Geometry check sheet. Reference: the model listing, model coordinates, mm. A direction names the side the tool comes from. Round coordinates to 2 decimals unless told otherwise and drop trailing zeros. Order: outer loops, then holes, each group sorted by start corner. A loop starts at its lowest first (then second) coordinate and runs counter-clockwise, first axis right, second up. Notation, with made-up numbers: (40.25, -18.75) -> (78.25, -18.75) arc R23 ccw to (78.25, 18.25) -> close; hole circle Ø5 at (59.25, 84.25). An arc over 180 degrees is marked (long way). Use a Markdown table: item, result. Add a question column.
Item 1: Mould release check, pull along Z, two halves, no side actions. Record for faces 1 (the flat face through (3, 0, 22)), 2 (the cylindrical face through (5.11, 0.31, 42.34)), 3 (the cylindrical face through (-2.648, 0.308, 9.225)), 4 (the cylindrical face through (-0.295, 0.308, -11.222)): pulls with the +Z half, pulls with the -Z half, needs draft (parallel to the pull), parting line crosses it, or undercut.
Item 2: Set-up check for faces 5 (the cylindrical face through (-6.117, 0.308, 73.465)), 6 (the cylindrical face through (-2.45, 0.31, 56.29)): record each of +Z, -Z, +X, -X, +Y, -Y from which the full face is reachable in a straight line by a thin tool's end or side.
Item 3: Sectioned sample at B-B, the plane y = 0.5. Record the cut outline in (x, z).
Item 4: Sectioned sample at D-D, the plane z = 53. Record the cut outline in (x, y) (3 decimals), and give its area (3 significant figures).
Item 5: Material ranges on probe 1 along Z at (x, y) = (-4, 0.2); probe 2 along Z at (x, y) = (-6.5, 0.4); probe 3 along X at (y, z) = (0.35, 36), recorded low to high. Write a range as [from, to].
Item 6: Sectioned sample at A-A, the plane x = -1.25. Record the cut outline in (y, z) (3 decimals), and give its area (3 significant figures).
Item 7: Sectioned sample at C-C, the plane x = -5. Record the cut outline in (y, z) (3 decimals).
from build123d import *

# Parameters (mm, degrees)
BOSS_EXTRUDE1_DEPTH = 0.625


with BuildPart() as part:
    # Sketch1 → Boss-Extrude1 (new body)
    with BuildSketch(Plane(origin=(0, 0, 0), x_dir=(1, 0, 0), z_dir=(0, 1, 0))):
        with BuildLine():
            Line((8.997858244, 2.423307145), (9.848841271, -36.576692855))
            ThreePointArc((9.848841271, -36.576692855), (9.449049837, -38.139678019), (8.297497314, -39.26958182))
            ThreePointArc((8.297497314, -39.26958182), (5.081486735, -42.390887707), (3.9, -46.714007366))
            Line((3.9, -46.714007366), (3.9, -73.714007366))
            ThreePointArc((3.9, -73.714007366), (2.934734568, -75.918515302), (0.660096509, -76.704399701))
            ThreePointArc((0.660096509, -76.704399701), (-6.19183571, -73.385709721), (-9, -66.309206939))
            ThreePointArc((-9, -66.309206939), (-2.386951858, -56.128417461), (-0.35, -44.160472472))
            Line((-0.35, -44.160472472), (-0.35, -16.910472472))
            ThreePointArc((-0.35, -16.910472472), (-2.711701155, -9.129084421), (-9, -3.97302682))
            Line((-9, -3.97302682), (-9, 2.22697318))
            ThreePointArc((-9, 2.22697318), (-0.098172823, 11.226437725), (8.997858244, 2.423307145))
        make_face()
    extrude(amount=BOSS_EXTRUDE1_DEPTH)


solid = part.part
Found:
| question | item | result |
|---|---|---|
| 1 | face 1 | needs draft |
| 1 | face 2 | pulls with the +Z half |
| 1 | face 3 | undercut |
| 1 | face 4 | pulls with the -Z half |
| 2 | face 5 | +Z, -X, +Y, -Y |
| 2 | face 6 | -X, +Y, -Y |
| 3 | outline | (-9, -2.23) arc R9 ccw to (9, -2.42) -> (9.85, 36.58) arc R3 ccw to (8.3, 39.27) arc R8.5 cw to (3.9, 46.71) -> (3.9, 73.71) arc R3 ccw to (0.66, 76.7) arc R10.5 ccw to (-9, 66.31) arc R30 cw to (-0.35, 44.16) -> (-0.35, 16.91) arc R14 cw to (-9, 3.97) -> close |
| 4 | outline | (-1.359, 0) -> (3.9, 0) -> (3.9, 0.625) -> (-1.359, 0.625) -> close |
| 4 | area | 3.29 mm2 |
| 5 | probe 1 | z = [-10.29, 7.48], [59.59, 75.18] |
| 5 | probe 2 | z = [-8.45, 5.32], [63.44, 73.04] |
| 5 | probe 3 | x = [-0.35, 9.84] |
| 6 | outline | (0, -11.14) -> (0.625, -11.14) -> (0.625, 11.972) -> (0, 11.972) -> close; (0, 52.582) -> (0.625, 52.582) -> (0.625, 76.372) -> (0, 76.372) -> close |
| 6 | area | 29.3 mm2 |
| 7 | outline | (0, -9.71) -> (0.625, -9.71) -> (0.625, 6.49) -> (0, 6.49) -> close; (0, 61.287) -> (0.625, 61.287) -> (0.625, 74.484) -> (0, 74.484) -> close |
